Autodesk Inventor part; units mm, degrees
ref_plane "Work Plane1" through (-17.5922, 0, 0) normal (0, -0.866, -0.5) x (1, 0, 0)
ref_plane "YZ Plane" through (0, 0, 0) normal (1, 0, 0) x (0, 1, 0)
ref_plane "XZ Plane" through (0, 0, 0) normal (0, 1, 0) x (-1, 0, 0)
sketch "Эскиз1" plane through (0, 0, 0) normal (1, 0, 0) x (0, 1, 0)
  line L0 (-9.2376, 0) -> (-4.6188, 8)
  line L1 (-4.6188, 8) -> (4.6188, 8)
  line L2 (4.6188, 8) -> (9.2376, 0)
  line L3 (9.2376, 0) -> (4.6188, -8)
  line L4 (4.6188, -8) -> (-4.6188, -8)
  line L5 (-4.6188, -8) -> (-9.2376, 0)
  point P0 (0, 0)
  point P1 (0, 0)
  dimension "d0" = 18.4752
extrude "Базовый элемент" add sketch "Эскиз1" along normal blind 8.4
sketch "Эскиз2" plane through (0, 0, 0) normal (0, 0, 1) x (1, 0, 0)
  line L0 (0, 4.6188) -> (0, 9.2376)
  line L1 (0, 9.2376) -> (8.4, 9.2376)
  line L2 (8.4, 4.6188) -> (8.4, 9.2376)
  line L3 (-1.68, 0) -> (10.08, 0)
  line L4 (1.11, 9.2376) -> (0, 7.315)
  line L5 (7.29, 9.2376) -> (8.4, 7.315)
  dimension "d3" = 30
  dimension "d4" = 30
  dimension "d5" = 14.63
  dimension "d6" = 14.63
revolve "Фаска1" cut sketch "Эскиз2" angle 360 about axis through (-10, 0, 0) along (1, 0, 0)
sketch "Эскиз3" plane through (8.4, 0, 0) normal (1, 0, 0) x (0, 0, -1)
  arc A0 (-0.625, -1.0825) -> (0.625, -1.0825) centre (0, 0) ccw
hole "Резьба" at (8.4, 0, 0) direction (-1, 0, 0) diameter 8.9175 end through all
chamfer "Фаска2" distance 0.5413 angle 30 1 edges at (8.4, 0, 4.4587) measured on face at (8.4, 6.2812, -0.7627)
chamfer "Фаска3" distance 0.5413 angle 30 1 edges at (0, 0, 4.4587) measured on face at (0, 6.2812, -0.7627)
ref_plane "Work Plane1" through (-17.5922, 0, 0) normal (0, -0.866, -0.5) x (1, 0, 0)
equation "\"d0\" = 1.1547 * SW"
equation "\"d1\" = KOH"
equation "\"d3\" = ANG1"
equation "\"d4\" = ANG2"
equation "\"d5\" = SW0"
equation "\"d6\" = SW01"
equation "\"d8\" = -0.5 * GD1 + 0.5 * NND"
equation "\"d40\" = -0.5 * GD1 + 0.5 * NND"
equation "\"d10\" = -0.5 * GD1 + 0.5 * NND"
equation "\"d41\" = -0.5 * GD1 + 0.5 * NND"
equation "\"ANG1\" = 30deg"
equation "\"ANG2\" = 30deg"
equation "\"KOH\" = 8.4"
equation "\"SW\" = 16"
equation "\"SW0\" = 14.63"
equation "\"SW01\" = SW0"
equation "\"GUL\" = 0.541266 * PTC"
equation "\"LADI\" = 12.345"
equation "\"TOA\" = 30deg"
equation "\"FAWI\" = 30deg"
equation "\"PTC\" = 1"
equation "\"E0\" = 1.155 * SW"
equation "\"GAL\" = 0.541266 * PTC"
properties part number "Копия гайки M10x1-6H ГОСТ 5915-70" material "Сталь, мягкая"
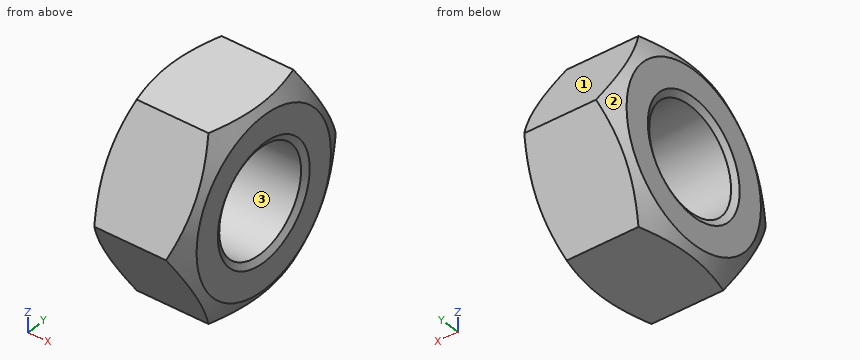
Input: part model. Units: mm. Frame: model coordinates. Face numbers are marked on the shaded views. Give positions to 0.01 mm unless a question says otherwise; leave off trailing zeros. Order: outer loops, then holes, each group sorted by start corner. A loop starts at its lowest first (then second) coordinate and runs counter-clockwise, first axis right, second up. Notation, with made-up numbers: M 88.25,3 L 95.25,3 A14 ccw 95.25,30 Z; hole C 72,20 d7. An arc over 180 degrees is marked long. Return JSON: item names as keys, results as strings.
Item 1: First-contact query: P1, Ø5, axis at x = 3, z = -4.5, coming from the -Y side; P2, Ø4, axis at x = 3.5, y = -7, coming from the +Z side; P3, Ø2, axis at y = 6.5, z = 5, coming from the +X side. Flat tips, straight axial feed; report the tip coordinate or a pass-through.
Solutions:
{"P1": "y = -8.08", "P2": "z = 7.34", "P3": "x = 8.4"}
Item 2: Cut plane B-B (x = 3). Return loops of the section in (y, z).
Solutions:
{"outline": "M -9.24,0 L -4.62,-8 L 4.62,-8 L 9.24,0 L 4.62,8 L -4.62,8 Z; hole C 0,0 d8.92"}
Item 3: Cut plane C-C (x = 7.5). Return loops of the section in (y, z), then the cut area to 3 significant figures.
Solutions:
{"outline": "M -8.85,-0.67 L -5.01,-7.33 A8.87 ccw -3.84,-8 L 3.84,-8 A8.87 ccw 5.01,-7.33 L 8.85,-0.67 A8.87 ccw 8.85,0.67 L 5.01,7.33 A8.87 ccw 3.84,8 L -3.84,8 A8.87 ccw -5.01,7.33 L -8.85,0.67 A8.87 ccw Z; hole C 0,0 d8.92", "area": "158 mm^2"}
Item 4: Ray query, probe 1 along Z at (x, y) = (3, 0); probe 2 along Y at (x, z) = (3.25, 2.5); probe 3 along Z at (x, y) = (1.75, -3.5). Return the intervals inside material, ascending.
Solutions:
{"probe 1": "-8 to -4.46, 4.46 to 8", "probe 2": "-7.79 to -3.69, 3.69 to 7.79", "probe 3": "-8 to -2.76, 2.76 to 8"}
Item 5: Pull-direction query (Y, two-part tool) for the marked faces 1, 2 and 3; classes: +Y half, -Y half, draft (parallel to the pull), parting line (faces both ways), or undercut.
Solutions:
{"face 1": "+Y half", "face 2": "parting line", "face 3": "undercut"}
Item 6: Cut plane A-A (y = 0). Return loops of the section in (x, z) (3 decimals).
Solutions:
{"outline": "M 0,-7.315 L 0.395,-8 L 8.005,-8 L 8.4,-7.315 L 8.4,-5 L 8.087,-4.459 L 0.313,-4.459 L 0,-5 Z; M 0,5 L 0.313,4.459 L 8.087,4.459 L 8.4,5 L 8.4,7.315 L 8.005,8 L 0.395,8 L 0,7.315 Z"}
